from build123d import *

# Parameters (mm, degrees)
SKETCH1_R           = 2.75
BOSS_EXTRUDE1_DEPTH = 4.7625


with BuildPart() as part:
    # Sketch1 → Boss-Extrude1 (new body)
    with BuildSketch(Plane.XY):
        with BuildLine():
            Line((-85, 0), (85, 0))
            Line((85, 0), (85, 40))
            Line((85, 40), (65, 40))
            ThreePointArc((65, 40), (0, 20.871205009), (-65, 40))
            Line((-65, 40), (-85, 40))
            Line((-85, 40), (-85, 0))
        make_face()
        with Locations((-75, 30)):
            Circle(SKETCH1_R, mode=Mode.SUBTRACT)
        with Locations((-75, 10)):
            Circle(SKETCH1_R, mode=Mode.SUBTRACT)
        with Locations((75, 30)):
            Circle(SKETCH1_R, mode=Mode.SUBTRACT)
        with Locations((75, 10)):
            Circle(SKETCH1_R, mode=Mode.SUBTRACT)
        with BuildLine():
            Line((-65, 23.206426932), (-65, 13))
            ThreePointArc((-65, 13), (-64.121320344, 10.878679656), (-62, 10))
            Line((-62, 10), (-36.578066235, 10))
            ThreePointArc((-36.578066235, 10), (-33.607128783, 12.583429889), (-35.752997072, 15.884312895))
            ThreePointArc((-35.752997072, 15.884312895), (-48.434787426, 20.230949012), (-60.601503759, 25.86051967))
            ThreePointArc((-60.601503759, 25.86051967), (-63.549921172, 25.775034407), (-65, 23.206426932))
        make_face(mode=Mode.SUBTRACT)
        with BuildLine():
            Line((65, 23.206426932), (65, 13))
            ThreePointArc((65, 13), (64.121320344, 10.878679656), (62, 10))
            Line((62, 10), (36.578066235, 10))
            ThreePointArc((36.578066235, 10), (33.607128783, 12.583429889), (35.752997072, 15.884312895))
            ThreePointArc((35.752997072, 15.884312895), (48.434787426, 20.230949012), (60.601503759, 25.86051967))
            ThreePointArc((60.601503759, 25.86051967), (63.549921172, 25.775034407), (65, 23.206426932))
        make_face(mode=Mode.SUBTRACT)
    extrude(amount=BOSS_EXTRUDE1_DEPTH)


solid = part.part
Geometry: final body of the model. Coordinates: model frame, mm. A direction names the side the tool comes from. Give positions to 0.01 mm unless a question says otherwise; leave off trailing zeros. Write each loop counter-clockwise with the first axis right and the second up, starting at its lowest first coordinate (ties: lowest second). Pieces come first, ordered by that corner, then holes. Notation, with made-up numbers: M 39.5,31.5 L 90.5,31.5 A26 cw 90.5,54.5 Z; hole C -10.75,-25 d3. An arc over 180 degrees is marked long. Answer in a Markdown table with one row per item. Add a question column.
(1) Section C-C on y = 35.5. Return loops of the section in (x, z).
(2) Mould query, pull axis Y, two halves, no side actions, for faces 3 (the flat face through (-75, 40, 2)), 4 (the flat face through (-49, 10, 2)), 5 (the flat face through (-1, 16, 0)). Classes: +Y half, -Y half, draft (parallel to the pull), parting line (faces both ways), or undercut.
(3) Section A-A on x = -75. Return loops of the section in (y, z).
(4) First-contact query: pin 1 (2 mm diameter, centred on x = -1.5, z = 1, fed in from -Y); pin 2 (1 mm diameter, centred on x = 12.5, z = 2.5, fed in from +Y); pin 3 (2.5 mm diameter, centred on x = -55.5, z = 2, fed in from +Y). Flat tips, straight axial feed; report the tip coordinate or a pass-through.
(5) Section D-D on x = 38. Return loops of the section in (y, z), and give its area (3 significant figures).
(6) Section B-B on z = 2.5. Return loops of the section in (x, y), and give its area (3 significant figures).
(7) Ray query, line 1 (Y direction, x = -75, z = 1.8); line 2 (X direction, y = 31, z = 3.6); line 3 (X direction, y = 20.5, z = 4.5). Return the intervals inside material, ascending.
(8) Reachability of faces 1 (the flat face through (85, 20, 2)), 2 (the flat face through (65, 18, 2)) from +Z, -Z, +X, -X, +Y, -Y: full face, straight path, thin tool, end or side. Return the list, or none.
Result set:
| question | item | result |
|---|---|---|
| 1 | outline | M -85,0 L -57.42,0 L -57.42,4.76 L -85,4.76 Z; M 57.42,0 L 85,0 L 85,4.76 L 57.42,4.76 Z |
| 2 | face 3 | +Y half |
| 2 | face 4 | undercut |
| 2 | face 5 | draft |
| 3 | outline | M 0,0 L 7.25,0 L 7.25,4.76 L 0,4.76 Z; M 12.75,0 L 27.25,0 L 27.25,4.76 L 12.75,4.76 Z; M 32.75,0 L 40,0 L 40,4.76 L 32.75,4.76 Z |
| 4 | pin 1 | stops at y = 0 |
| 4 | pin 2 | stops at y = 21.58 |
| 4 | pin 3 | stops at y = 35.14 |
| 5 | outline | M 0,0 L 10,0 L 10,4.76 L 0,4.76 Z; M 16.55,0 L 27.05,0 L 27.05,4.76 L 16.55,4.76 Z |
| 5 | area | 97.6 mm^2 |
| 6 | outline | M -85,0 L 85,0 L 85,40 L 65,40 A120 cw -65,40 L -85,40 Z; hole C -75,10 d5.5; hole C -75,30 d5.5; hole M -65,13 A3 ccw -62,10 L -36.58,10 A3 ccw -35.75,15.88 A130 cw -60.6,25.86 A3 ccw -65,23.21 Z; hole M 35.75,15.88 A3 ccw 36.58,10 L 62,10 A3 ccw 65,13 L 65,23.21 A3 ccw 60.6,25.86 A130 cw Z; hole C 75,10 d5.5; hole C 75,30 d5.5 |
| 6 | area | 4,350 mm^2 |
| 7 | line 1 | y = 0 to 7.25, 12.75 to 27.25, 32.75 to 40 |
| 7 | line 2 | x = -85 to -77.56, -72.44 to -48.25, 48.25 to 72.44, 77.56 to 85 |
| 7 | line 3 | x = -85 to -65, -49.1 to 49.1, 65 to 85 |
| 8 | face 1 | +Z, -Z, +X, +Y, -Y |
| 8 | face 2 | +Z, -Z |
